```python
from build123d import *

# Parameters (mm, degrees)
SKETCH_1_W          = 60
SKETCH_1_H          = 30
EXTRUDE_1_DEPTH     = 4
SKETCH_2_R          = 1.5
CUT_EXTRUDE_1_DEPTH = 4
SKETCH_3_R          = 11.5
CUT_EXTRUDE_2_DEPTH = 4
SKETCH_4_R          = 1.5
CUT_EXTRUDE_3_DEPTH = 4
FILLET_1_R          = 5


with BuildPart() as part:
    # 草图1 → 凸台-拉伸1 (new body)
    with BuildSketch(Plane(origin=(0, 0, 0), x_dir=(1, 0, 0), z_dir=(0, 1, 0))):
        Rectangle(SKETCH_1_W, SKETCH_1_H)
    extrude(amount=EXTRUDE_1_DEPTH)

    # 草图2 → 切除-拉伸1 (cut)
    with BuildSketch(Plane(origin=(0, 4, 0), x_dir=(1, 0, 0), z_dir=(0, 1, 0))):
        with Locations(Location((-24, 5, 0), (0, 0, 270))):
            Circle(SKETCH_2_R)
        with Locations(Location((-24, -5, 0), (0, 0, 270))):
            Circle(SKETCH_2_R)
        with Locations(Location((24, -5, 0), (0, 0, 270))):
            Circle(SKETCH_2_R)
        with Locations(Location((24, 5, 0), (0, 0, 270))):
            Circle(SKETCH_2_R)
    extrude(amount=-CUT_EXTRUDE_1_DEPTH, mode=Mode.SUBTRACT)

    # 草图3 → 切除-拉伸2 (cut)
    with BuildSketch(Plane(origin=(0, 4, 0), x_dir=(1, 0, 0), z_dir=(0, 1, 0))):
        with Locations(Location((10, 0, 0), (0, 0, 270))):
            Circle(SKETCH_3_R)
    extrude(amount=-CUT_EXTRUDE_2_DEPTH, mode=Mode.SUBTRACT)

    # 草图4 → 切除-拉伸3 (cut)
    with BuildSketch(Plane(origin=(0, 4, 0), x_dir=(1, 0, 0), z_dir=(0, 1, 0))):
        with Locations(Location((-12, 0, 0), (0, 0, 270))):
            Circle(SKETCH_4_R)
    extrude(amount=-CUT_EXTRUDE_3_DEPTH, mode=Mode.SUBTRACT)

    # 圆角1
    fillet_1_edges = [part.edges().sort_by_distance(p)[0] for p in [
        (30, 2, 15),
        (-30, 2, 15),
        (-30, 2, -15),
        (30, 2, -15),
    ]]
    fillet(fillet_1_edges, radius=FILLET_1_R)


solid = part.part
```
Geometry: final body of the model. Coordinates: model frame, mm. Round coordinates to 2 decimals unless told otherwise and drop trailing zeros. Order: outer loops, then holes, each group sorted by start corner. A loop starts at its lowest first (then second) coordinate and runs counter-clockwise, first axis right, second up. Notation, with made-up numbers: (-3, -18.75) - (24, -18.75) arc R14 cw to (24, -14.75) - close; hole circle Ø8 at (-4, 55). An arc over 180 degrees is marked (long way). Write item = value, one per line. Start each with the question number.
Q1. Cut plane D-D on y = 1.75. Return the cut outline in (x, z), and give its area (3 significant figures).
Q2. Pin query (flat end, axial travel): pin 1 (2.5 mm diameter, centred on x = 24, z = -5, fed in from +Y). Return the tip coordinate at first contact, or that it passes through.
Q3. Cut plane B-B on z = 0. Return the cut outline in (x, y), and give its area (3 significant figures).
Q4. Ray query, line 1 (X direction, y = 1.25, z = 5); line 2 (Z direction, x = 25, y = 2.15); line 3 (X direction, y = 0.5, z = -5.75). Return the intervals inside material, ascending. Write a range as from..to.
Q5. Pull-direction query (X, two-part tool) for faces 1 (the cylindrical face through (-11.55, 2.03, 1.43)), 2 (the flat face through (0, 2, -15)), 3 (the cylindrical face through (28, 2, 14)); classes: +X half, -X half, draft (parallel to the pull), parting line (faces both ways), or undercut.
Q6. Cut plane A-A on x = 10. Return the cut outline in (y, z), and give its area (3 significant figures).
Q7. Cut plane C-C on x = 24. Return the cut outline in (y, z), and give its area (3 significant figures).
Outcome:
q1.outline = (-30, -10) arc R5 ccw to (-25, -15) - (25, -15) arc R5 ccw to (30, -10) - (30, 10) arc R5 ccw to (25, 15) - (-25, 15) arc R5 ccw to (-30, 10) - close; hole circle Ø3 at (-24, -5); hole circle Ø3 at (-24, 5); hole circle Ø3 at (-12, 0); hole circle Ø23 at (10, 0); hole circle Ø3 at (24, -5); hole circle Ø3 at (24, 5)
q1.area = 1,330 mm^2
q2.pin_1 = through
q3.outline = (-30, 0) - (-13.5, 0) - (-13.5, 4) - (-30, 4) - close; (-10.5, 0) - (-1.5, 0) - (-1.5, 4) - (-10.5, 4) - close; (21.5, 0) - (30, 0) - (30, 4) - (21.5, 4) - close
q3.area = 136 mm^2
q4.line_1 = -30..-25.5, -22.5..-0.36, 20.36..22.5, 25.5..30
q4.line_2 = -15..-6.12, -3.88..3.88, 6.12..15
q4.line_3 = -30..-25.3, -22.7..0.04, 19.96..22.7, 25.3..30
q5.face_1 = undercut
q5.face_2 = draft
q5.face_3 = +X half
q6.outline = (0, -15) - (4, -15) - (4, -11.5) - (0, -11.5) - close; (0, 11.5) - (4, 11.5) - (4, 15) - (0, 15) - close
q6.area = 28.0 mm^2
q7.outline = (0, -15) - (4, -15) - (4, -6.5) - (0, -6.5) - close; (0, -3.5) - (4, -3.5) - (4, 3.5) - (0, 3.5) - close; (0, 6.5) - (4, 6.5) - (4, 15) - (0, 15) - close
q7.area = 96.0 mm^2
